Autodesk Fusion 360 part; units mm, degrees
sketch "Sketch1" plane through (0, 0, 0) normal (0, 0, 1) x (1, 0, 0)
  line L0 (0, 0) -> (16.5, 0)
  line L1 (16.5, 0) -> (16.5, 19.43)
  line L2 (16.5, 19.43) -> (0, 19.43)
  line L3 (0, 19.43) -> (0, 0)
  line L4 (0, 19.43) -> (1.2, 19.43)
  line L5 (1.2, 0) -> (0, 0)
  line L6 (0, 0) -> (0, 19.43)
  line L7 (16.5, 19.43) -> (13.5, 19.43)
  line L8 (13.5, 19.43) -> (13.5, 0)
  line L9 (13.5, 0) -> (16.5, 0)
  line L10 (16.5, 0) -> (16.5, 19.43)
  line L11 (-4.4, -5.285) -> (21.9, -5.285)
  line L12 (21.9, -5.285) -> (21.9, 24.715)
  line L13 (21.9, 24.715) -> (-4.4, 24.715)
  line L14 (-4.4, 24.715) -> (-4.4, -5.285)
  line L15 (0, 0) -> (13.5, 0)
  line L16 (13.5, 0) -> (13.5, 0.75)
  line L17 (13.5, 0.75) -> (0, 0.75)
  line L18 (0, 0.75) -> (0, 0)
  line L19 (0, 19.43) -> (13.5, 19.43)
  line L20 (13.5, 19.43) -> (13.5, 18.68)
  line L21 (13.5, 18.68) -> (0, 18.68)
  line L22 (0, 18.68) -> (0, 19.43)
  line L23 (-2.55, -3.435) -> (20.05, -3.435)
  line L24 (20.05, -3.435) -> (20.05, 22.865)
  line L25 (20.05, 22.865) -> (-2.55, 22.865)
  line L26 (-2.55, 22.865) -> (-2.55, -3.435)
  dimension "d1" = 16.5
  dimension "d2" = 19.43
  dimension "d4" = 3
  dimension "d9" = 4.4
  dimension "d49" = 0.75
  dimension "d50" = 0.75
  dimension "d53" = 30
  dimension "d54" = 5.285
  dimension "d55" = 1.85
  dimension "d56" = 1.85
  dimension "d57" = 1.85
  dimension "d58" = 1.85
  dimension "d71" = 5.4
  dimension "d72" = 25.3
extrude "Extrude14" add sketch "Sketch1" along normal blind 1.62 contours L11 L12 L13 L14
extrude "Extrude15" add sketch "Sketch1" against normal blind 3.38 contours L11 L12 L13 L14
extrude "Extrude16" add sketch "Sketch1" against normal blind 1.38 contours L0 L3 L5 L6 L8 L15 L16 L17 L18 | L0 L1 L2 L7 L8 L9 L10 L16 L20 | L2 L3 L4 L6 L8 L19 L20 L21 L22 | L23 L24 L25 L26
equation "d32 = ( 16.50 mm - d27 ) / 2"
equation "d49 = d50"
equation "d54 = ( d53 - d2 ) / 2"
equation "d56 = d55"
equation "d57 = d55"
equation "d58 = d55"
Check sheet for the modelled part. Datum: model origin and axes. Units: mm. A direction names the side the tool comes from. Round coordinates to 2 decimals unless told otherwise and drop trailing zeros. Order: outer loops, then holes, each group sorted by start corner. A loop starts at its lowest first (then second) coordinate and runs counter-clockwise, first axis right, second up.
(1) Cross-section at A-A, the plane z = -0.8. Enter the section's corners in (x, y) (3 decimals), and give its area (3 significant figures).
(2) Scan lines: probe 1 along X at (y, z) = (11.5, -2.65); probe 2 along X at (y, z) = (10.75, -1.2); probe 3 along Y at (x, z) = (-2.5, -2.8) (3 decimals). Record each from-to range of solid material in increasing order.
(3) Cross-section at C-C, the plane x = 11. Enter the section's corners in (y, z) (3 decimals), and give its area (3 significant figures).
(4) Cross-section at B-B, the plane y = 17. Enter the section's corners in (x, z).
(5) Cross-section at D-D, the plane x = 16.5. Enter the section's corners in (y, z) (3 decimals).
(6) Access from +Z, -Z, +X, -X, +Y, -Y to the whole of each face (thin tool, end or side, straight path). Record for faces 1 (the flat face through (9, -5.285, -1)), 2 (the flat face through (-3, 10, -3.38)), 3 (the flat face through (-2.55, 10, -2)), 4 (the flat face through (9, 22.865, 1)), 5 (the flat face through (7, 0.75, -1)).
(7) Go/stop test with a flat-tipped pin: P1, Ø1, axis at x = 19, y = 13, coming from the -Z side. Record where the tip stops, or that it passes through.
(8) Draft check along Y on faces 6 (the flat face through (9, -3.435, 1)), 7 (the flat face through (21.9, 10, -1)), 8 (the flat face through (9, 24.715, -1)). Enter one of: pulls with the +Y half, pulls with the -Y half, needs draft (parallel to the pull), parting line crosses it, or undercut.
Check sheet entries:
1. outline: (-4.4, -5.285) - (21.9, -5.285) - (21.9, 24.715) - (-4.4, 24.715) - close; hole (0, 0.75) - (13.5, 0.75) - (13.5, 18.68) - (0, 18.68) - close
1. area: 547 mm2
2. probe 1: x = -4.4 to -2.55, 20.05 to 21.9
2. probe 2: x = -4.4 to 0, 13.5 to 21.9
2. probe 3: y = -5.285 to -3.435, 22.865 to 24.715
3. outline: (-5.285, -3.38) - (-3.435, -3.38) - (-3.435, -1.38) - (0.75, -1.38) - (0.75, 0) - (-3.435, 0) - (-3.435, 1.62) - (-5.285, 1.62) - close; (18.68, -1.38) - (22.865, -1.38) - (22.865, -3.38) - (24.715, -3.38) - (24.715, 1.62) - (22.865, 1.62) - (22.865, 0) - (18.68, 0) - close
3. area: 30.1 mm2
4. outline: (-4.4, -3.38) - (-2.55, -3.38) - (-2.55, -1.38) - (0, -1.38) - (0, 0) - (-2.55, 0) - (-2.55, 1.62) - (-4.4, 1.62) - close; (13.5, -1.38) - (20.05, -1.38) - (20.05, -3.38) - (21.9, -3.38) - (21.9, 1.62) - (20.05, 1.62) - (20.05, 0) - (13.5, 0) - close
5. outline: (-5.285, -3.38) - (-3.435, -3.38) - (-3.435, -1.38) - (22.865, -1.38) - (22.865, -3.38) - (24.715, -3.38) - (24.715, 1.62) - (22.865, 1.62) - (22.865, 0) - (-3.435, 0) - (-3.435, 1.62) - (-5.285, 1.62) - close
6. face 1: +Z, -Z, +X, -X, -Y
6. face 2: -Z, +X, -X, +Y, -Y
6. face 3: -Z
6. face 4: +Z
6. face 5: +Z, -Z
7. P1: stops at z = -1.38
8. face 6: undercut
8. face 7: needs draft
8. face 8: pulls with the +Y half
